```python
from build123d import *

# Parameters (mm, degrees)
F1_DEPTH = 15
F2_R     = 2.25
F3_DEPTH = 25
F4_R     = 2.25
F5_DEPTH = 5
F6_SIZE  = 1.5
F8_DEPTH = 1.5
F9_R     = 1


with BuildPart() as f1:
    # F0 (on Front) → F1 (new body)
    with BuildSketch(Plane.XZ):
        Polygon((-57.5, -25.5), (-57.5, 25.5), (-8.5, 25.5), (-2.5, 25.5), (-2.5, 41.5), (-8.5, 41.5), (-8.5, 29.5), (-61.5, 29.5), (-61.5, -29.5), (61.5, -29.5), (61.5, 29.5), (8.5, 29.5), (8.5, 41.5), (2.5, 41.5), (2.5, 25.5), (8.5, 25.5), (57.5, 25.5), (57.5, -25.5), align=None)
    extrude(amount=F1_DEPTH)

    # F2 (on face) → F3 (cut)
    with BuildSketch(Plane.YZ.offset(8.5)):
        with Locations((-7.5, 35.5)):
            Circle(F2_R)
    extrude(amount=-F3_DEPTH, mode=Mode.SUBTRACT)

    # F4 (on face) → F5 (cut)
    with BuildSketch(Plane(origin=(0, 0, -29.5), x_dir=(1, 0, 0), z_dir=(0, 0, -1))):
        with Locations((-42.25, 7.5)):
            Circle(F4_R)
        with Locations((42.25, 7.5)):
            Circle(F4_R)
    extrude(amount=-F5_DEPTH, mode=Mode.SUBTRACT)

    # F6
    f6_edges = [f1.edges().sort_by_distance(p)[0] for p in [
        (-44.5, -7.5, -25.5),
        (40, -7.5, -25.5),
    ]]
    chamfer(f6_edges, length=F6_SIZE)

    # F7 (on face) → F8 (cut)
    with BuildSketch(Plane(origin=(-8.5, 0, 0), x_dir=(0, -1, 0), z_dir=(-1, 0, 0))):
        Polygon((9.457997, 31.964525), (11.540809, 35.427938), (9.582812, 38.963412), (5.542003, 39.035475), (3.459191, 35.572062), (5.417188, 32.036588), align=None)
    extrude(amount=-F8_DEPTH, mode=Mode.SUBTRACT)

    # F9
    f9_edges = [f1.edges().sort_by_distance(p)[0] for p in [
        (30, 0, 25.5),
        (57.5, 0, 0),
        (-30, 0, 25.5),
        (-57.5, 0, 0),
        (0, 0, -25.5),
        (-30, -15, 25.5),
        (30, -15, 25.5),
        (-57.5, -15, 0),
        (0, -15, -25.5),
        (57.5, -15, 0),
    ]]
    fillet(f9_edges, radius=F9_R)


solid = f1.part
```
Source: CAD feature listing. Evaluate the final solid. Frame: model axes, mm. A direction names the side the tool comes from. Coordinates: 2 decimals unless noted, no trailing zeros. Write each loop counter-clockwise with the first axis right and the second up, starting at its lowest first coordinate (ties: lowest second). Pieces come first, ordered by that corner, then holes. Notation, with made-up numbers: (7.25, 32.5) -> (54.25, 32.5) arc R19 ccw to (54.25, 48.5) -> close; hole circle Ø10 at (36, 87). An arc over 180 degrees is marked (long way). Return JSON: item names as keys, results as strings. Group by question number.
1) Section query A-A, the plane z = -1. Return loops of the section in (x, y).
2) Contact query for flat-ended pins moving along their axis: P1, Ø5, axis at y = -7.5, z = 35.5, coming from the +X side; P2, Ø1.5, axis at x = 0.5, y = -10.5, coming from the +Z side; P3, Ø4.5, axis at y = -4.5, z = 34, coming from the -X side. Output: stop coordinate, or through.
3) Section query C-C, the plane y = -7.5. State how many separate pieces and enclosed holes the cut face has, plus the area to 3 significant figures.
4) Section query B-B, the plane x = -42.25. Return loops of the section in (y, z), plus the area to 3 significant figures.
5) Mould query, pull axis Z, two halves, no side actions, for faces 1 (the face through (30, -7, 25.5)), 2 (the face through (-5, -7, 41.5)), 3 (the face through (-1, -7, -29.5)). Classes: +Z half, -Z half, draft (parallel to the pull), parting line (faces both ways), or undercut.
6) Set-up query: faces 4 (the face through (-30, -7, 25.5)), 5 (the face through (-7, -7, 33)), 6 (the face through (8.5, -7, 33)). Return all of +Z, -Z, +X, -X, +Y, -Y with unobstructed straight access to the full face (end or side cutting, diameter ignored); none if empty.
7) Ray query, line 1 along X through (y, z) = (-7.5, -28.35); line 2 along Z through (x, y) = (-4.9, -7.5); line 3 along X through (y, z) = (-4.5, 32). Return the intervals inside material, ascending.
From the geometry:
{
 "1": {"outline": "(-61.5, -15) -> (-58.5, -15) arc R1 ccw to (-57.5, -14) -> (-57.5, -1) arc R1 ccw to (-58.5, 0) -> (-61.5, 0) -> close; (57.5, -14) arc R1 ccw to (58.5, -15) -> (61.5, -15) -> (61.5, 0) -> (58.5, 0) arc R1 ccw to (57.5, -1) -> close"},
 "2": {"P1": "x = 8.5", "P2": "z = -25.5", "P3": "x = -8.5"},
 "3": {"separate pieces": "5", "enclosed holes": "0", "area": "1,420 mm²"},
 "4": {"outline": "(-15, -29.5) -> (-9.75, -29.5) -> (-9.75, -27) -> (-11.25, -25.5) -> (-14, -25.5) arc R1 ccw to (-15, -26.5) -> close; (-15, 26.5) arc R1 ccw to (-14, 25.5) -> (-1, 25.5) arc R1 ccw to (0, 26.5) -> (0, 29.5) -> (-15, 29.5) -> close; (-5.25, -29.5) -> (0, -29.5) -> (0, -26.5) arc R1 ccw to (-1, -25.5) -> (-3.75, -25.5) -> (-5.25, -27) -> close", "area": "98.9 mm²"},
 "5": {"face 1": "undercut", "face 2": "+Z half", "face 3": "-Z half"},
 "6": {"face 4": "+Y, -Y", "face 5": "-X", "face 6": "+Z, +X, +Y, -Y"},
 "7": {"line 1": "-61.5 to -44.5, -40 to 40, 44.5 to 61.5", "line 2": "-29.5 to -25.5, 25.5 to 33.25, 37.75 to 41.5", "line 3": "-8.5 to -2.5, 2.5 to 8.5"}
}
